For this review, take the finished solid that the model builds, in its own axes (mm). Face numbers are marked on the shaded views. A direction names the side the tool comes from. Coordinates: 2 decimals unless noted, no trailing zeros. Loops run counter-clockwise (first coordinate to the right, second up) from the corner with the lowest first, then second, coordinate; pieces in that order, holes last. Notation, with made-up numbers: (41.25, 75) -> (99.25, 75) arc R32 cw to (99.25, 101) -> close; hole circle Ø5 at (3.5, -6.5). An arc over 180 degrees is marked (long way). Answer in a Markdown table with one row per item.
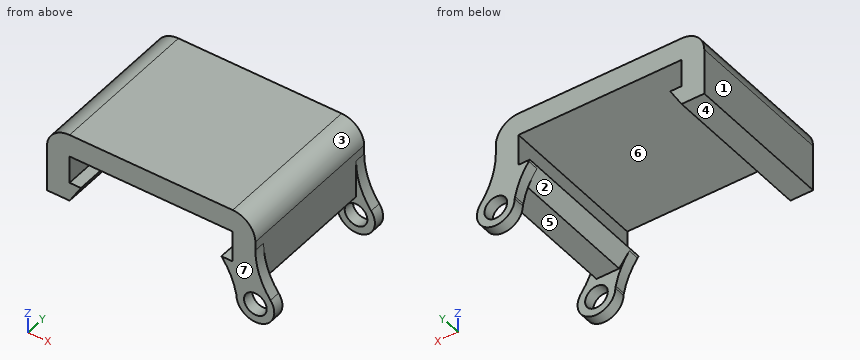
from build123d import *

# Parameters (mm, degrees)
SKETCH1_W           = 27.59
SKETCH1_H           = 20
BOSS_EXTRUDE1_DEPTH = 3
SKETCH2_W           = 3
SKETCH2_H           = 20
BOSS_EXTRUDE2_DEPTH = 6.175
BOSS_EXTRUDE3_DEPTH = 20
BOSS_EXTRUDE5_DEPTH = 1.5
BOSS_EXTRUDE6_START = -1.5
BOSS_EXTRUDE6_DEPTH = 1.5
CUT_EXTRUDE1_START  = -20
SKETCH8_R           = 1.5
CUT_EXTRUDE1_DEPTH  = 20
FILLET1_R           = 10
FILLET2_R           = 10
FILLET4_R           = 3


with BuildPart() as part:
    # Sketch1 → Boss-Extrude1 (new body)
    with BuildSketch(Plane.XY.offset(24.175)):
        with Locations((0, 65.784687602)):
            Rectangle(SKETCH1_W, SKETCH1_H)
    extrude(amount=BOSS_EXTRUDE1_DEPTH)

    # Sketch2 → Boss-Extrude2 (add)
    with BuildSketch(Plane(origin=(0, 0, 24.175), x_dir=(-1, 0, 0), z_dir=(0, 0, -1))):
        with Locations((-12.295, 65.784687602)):
            Rectangle(SKETCH2_W, SKETCH2_H)
        with Locations((12.295, 65.784687602)):
            Rectangle(SKETCH2_W, SKETCH2_H)
    extrude(amount=BOSS_EXTRUDE2_DEPTH)

    # Sketch4 → Boss-Extrude3 (add)
    with BuildSketch(Plane(origin=(0, 75.784687602, 0), x_dir=(1, 0, 0), z_dir=(0, 1, 0))):
        Polygon((-10.795, -20.5), (-10.795, -18), (-9.295, -20.5), align=None)
        Polygon((10.795, -18), (10.795, -20), (9.295, -20), align=None)
    extrude(amount=-BOSS_EXTRUDE3_DEPTH)

    # Sketch6 → Boss-Extrude5 (add)
    with BuildSketch(Plane.XZ.offset(-55.784687602)):
        with BuildLine():
            Line((10.795, 18), (11.295, 15.5))
            ThreePointArc((11.295, 15.5), (15.562766953, 13.732233047), (13.795, 18))
            Line((13.795, 18), (10.795, 18))
        make_face()
    extrude(amount=-BOSS_EXTRUDE5_DEPTH)

    # Sketch7 → Boss-Extrude6 (add)
    with BuildSketch(Plane(origin=(0, 75.784687602, 0), x_dir=(1, 0, 0), z_dir=(0, 1, 0)).offset(BOSS_EXTRUDE6_START)):
        with BuildLine():
            Line((10.795, -18), (11.295, -15.5))
            ThreePointArc((11.295, -15.5), (15.562766953, -13.732233047), (13.795, -18))
            Line((13.795, -18), (10.795, -18))
        make_face()
    extrude(amount=BOSS_EXTRUDE6_DEPTH)

    # Sketch8 → Cut-Extrude1 (cut)
    with BuildSketch(Plane(origin=(0, 75.784687602, 0), x_dir=(1, 0, 0), z_dir=(0, 1, 0)).offset(CUT_EXTRUDE1_START)):
        with Locations(Location((13.795, -15.5, 0), (0, 0, 270))):
            Circle(SKETCH8_R)
    extrude(amount=CUT_EXTRUDE1_DEPTH, mode=Mode.SUBTRACT)

    # Fillet1
    fillet1_edges = [part.edges().sort_by_distance(p)[0] for p in [
        (13.795, 75.034687602, 18),
        (13.795, 56.534687602, 18),
    ]]
    fillet(fillet1_edges, radius=FILLET1_R)

    # Fillet2
    fillet2_edges = [part.edges().sort_by_distance(p)[0] for p in [
        (10.795, 56.534687602, 18),
        (10.795, 75.034687602, 18),
    ]]
    fillet(fillet2_edges, radius=FILLET2_R)

    # Fillet4
    fillet4_edges = [part.edges().sort_by_distance(p)[0] for p in [
        (13.795, 65.784687602, 27.175),
        (-13.795, 65.784687602, 27.175),
    ]]
    fillet(fillet4_edges, radius=FILLET4_R)


solid = part.part
Item 1: The part is to be moulded in two halves that separate along X. For the marked faces 1, 2 and 3, say which applies: +X half, -X half, draft (parallel to the pull), parting line (faces both ways), or undercut.
Worked answers:
| item | result |
|---|---|
| face 1 | -X half |
| face 2 | undercut |
| face 3 | +X half |
Item 2: Insertion check: pin 1 (1.5 mm diameter, centred on x = 12.5, y = 62, fed in from -Z); pin 2 (4 mm diameter, centred on y = 63.5, z = 20.5, fed in from +X) (3 decimals); pin 3 (10 mm diameter, centred on x = -3.5, y = 67.5, fed in from -Z) (3 decimals). Each pin has a flat end and moves straight along its axis. Give the tip position at first contact, or say it passes through.
Worked answers:
| item | result |
|---|---|
| pin 1 | z = 18 |
| pin 2 | x = 13.795 |
| pin 3 | z = 24.175 |
Item 3: Take a section at D-D, the plane x = -3.5. State the section outline as (y, z) points (3 decimals).
Worked answers:
| item | result |
|---|---|
| outline | (55.785, 24.175) -> (75.785, 24.175) -> (75.785, 27.175) -> (55.785, 27.175) -> close |
Item 4: Take a section at A-A, the plane z = 23.5. State the section outline as (x, y) points (3 decimals), and give its area (3 significant figures).
Worked answers:
| item | result |
|---|---|
| outline | (-13.795, 55.785) -> (-10.795, 55.785) -> (-10.795, 75.785) -> (-13.795, 75.785) -> close; (10.795, 55.785) -> (13.795, 55.785) -> (13.795, 75.785) -> (10.795, 75.785) -> close |
| area | 120 mm² |
Item 5: Take a section at C-C, the plane y = 63.5. State the section outline as (x, z) points (3 decimals).
Worked answers:
| item | result |
|---|---|
| outline | (-13.795, 18) -> (-10.795, 18) -> (-9.295, 20.5) -> (-10.795, 20.5) -> (-10.795, 24.175) -> (10.795, 24.175) -> (10.795, 20) -> (9.295, 20) -> (10.795, 18) -> (13.795, 18) -> (13.795, 24.175) arc R3 ccw to (10.795, 27.175) -> (-10.795, 27.175) arc R3 ccw to (-13.795, 24.175) -> close |
Item 6: For L1, parallel to X at y = 74.9, z = 15.5 (3 decimals); L2, parallel to X at y = 68.5, z = 24 (3 decimals); L3, parallel to Z at x = 1, y = 59.5 (3 decimals), list the stretches that pass through material, from the lowest coordinate up.
Worked answers:
| item | result |
|---|---|
| L1 | 11.295 to 12.295, 15.295 to 16.295 |
| L2 | -13.795 to -10.795, 10.795 to 13.795 |
| L3 | 24.175 to 27.175 |
Item 7: Take a section at B-B, the plane x = 10. State the section outline as (y, z) points (3 decimals), and give its area (3 significant figures).
Worked answers:
| item | result |
|---|---|
| outline | (55.785, 18.974) -> (57.285, 18.974) -> (57.285, 19.06) -> (74.285, 19.06) -> (74.285, 18.974) -> (75.785, 18.974) -> (75.785, 20) -> (55.785, 20) -> close; (55.785, 24.175) -> (75.785, 24.175) -> (75.785, 27.175) -> (55.785, 27.175) -> close |
| area | 79.1 mm² |
Item 8: For the marked faces 4, 5, 6 and 7, list the 3-axis set-ups (+Z, -Z, +X, -X, +Y, -Y) from which the entire face can be reached by the end or side of a thin tool; tool diameter is ignored.
Worked answers:
| item | result |
|---|---|
| face 4 | -Z, -X, +Y, -Y |
| face 5 | -Z, +X, -X |
| face 6 | +Y, -Y |
| face 7 | +Z, -Z, +X, -X, -Y |
